Check sheet for the modelled part. Datum: model origin and axes. Units: mm. Face numbers are marked on the shaded views. A direction names the side the tool comes from. Give positions to 0.01 mm unless a question says otherwise; leave off trailing zeros. Order: outer loops, then holes, each group sorted by start corner. A loop starts at its lowest first (then second) coordinate and runs counter-clockwise, first axis right, second up.
Item 1: Sectioned sample at C-C on y = 5. Record the boundary of the cut face in (x, z), and give its area (3 significant figures).
Item 2: Sectioned sample at D-D on x = 7.5. Record the boundary of the cut face in (y, z), and give its area (3 significant figures).
Item 3: Material ranges on line 1 along X through (y, z) = (0, -80); line 2 along X through (y, z) = (0, -74.5); line 3 along Z through (x, y) = (3, 14), recorded low to high.
Item 4: Sectioned sample at A-A on y = 0. Record the boundary of the cut face in (x, z), and give its area (3 significant figures).
Item 5: Release check for a two-part mould opening along Y. For the marked faces 4, 5 and 6 record: released by +Y, released by -Y, zero draft, split by the parting line, or undercut.
Item 6: Gauge pin test, flat ends, axial feed: P1, Ø1, axis at x = 5.5, z = -73.5, coming from the +Y side; P2, Ø3, axis at x = 0.5, z = -78.5, coming from the -Y side; P3, Ø2, axis at x = 12.5, y = 16, coming from the -Z side. Record the tip position at first contact, or that the pin passes through.
Item 7: Access from +Z, -Z, +X, -X, +Y, -Y to the whole of each face (thin tool, end or side, straight path). Record for the marked faces 1, 2 and 3.
Autodesk Inventor part; units mm, degrees
ref_plane "YZ Plane" through (0, 0, 0) normal (1, 0, 0) x (0, 1, 0)
ref_plane "XZ Plane" through (0, 0, 0) normal (0, 1, 0) x (-1, 0, 0)
ref_plane "XY Plane" through (0, 0, 0) normal (0, 0, 1) x (1, 0, 0)
sketch "Sketch1" plane through (0, 0, 0) normal (1, 0, 0) x (0, 1, 0)
  line L0 (0, 0) -> (2.5, 0)
  line L1 (0, 0) -> (4, 0)
  line L2 (2.5, 0) -> (2.5, -7)
  line L3 (2.5, -7) -> (0, -7)
  line L4 (0, -7) -> (20, -7)
  line L5 (4, 0) -> (4, -7)
  line L6 (2.5, -7) -> (2.5, -41)
  line L7 (20, -7) -> (20, -11)
  line L8 (20, -11) -> (2.5, -11)
  line L9 (20, -7) -> (22.5, -7)
  line L10 (22.5, -7) -> (22.5, -11)
  line L11 (22.5, -11) -> (20, -11)
  line L12 (20, -11) -> (20, -7)
  line L13 (20, -7) -> (20, -11)
  line L14 (4, 0) -> (2.5, 0)
  line L15 (2.5, 0) -> (2.5, -11)
  line L16 (2.5, -11) -> (4, -11)
  line L17 (4, -11) -> (4, 0)
  line L18 (2.5, -11) -> (22.5, -11)
  line L19 (22.5, -11) -> (22.5, -7)
  line L20 (22.5, -7) -> (2.5, -7)
  line L21 (2.5, -7) -> (2.5, -11)
  line L22 (2.5, -11) -> (6.5, -11)
  line L23 (0, -7) -> (0, -105.9451)
  line L24 (2.5, -41) -> (25, -41)
  line L25 (0, -82) -> (2.5, -82)
  line L26 (0, -82) -> (4, -82)
  line L27 (2.5, -82) -> (2.5, -75)
  line L28 (2.5, -75) -> (0, -75)
  line L29 (0, -75) -> (20, -75)
  line L30 (4, -82) -> (4, -75)
  line L31 (20, -75) -> (20, -71)
  line L32 (20, -71) -> (2.5, -71)
  line L33 (20, -75) -> (22.5, -75)
  line L34 (22.5, -75) -> (22.5, -71)
  line L35 (22.5, -71) -> (20, -71)
  line L36 (20, -71) -> (20, -75)
  line L37 (20, -75) -> (20, -71)
  line L38 (4, -82) -> (2.5, -82)
  line L39 (2.5, -82) -> (2.5, -71)
  line L40 (2.5, -71) -> (4, -71)
  line L41 (4, -71) -> (4, -82)
  line L42 (2.5, -71) -> (22.5, -71)
  line L43 (22.5, -71) -> (22.5, -75)
  line L44 (22.5, -75) -> (2.5, -75)
  line L45 (2.5, -75) -> (2.5, -71)
  line L46 (2.5, -71) -> (6.5, -71)
  line L47 (2.5, -11) -> (6.5, -11)
  line L48 (6.5, -11) -> (6.5, -71)
  line L49 (6.5, -71) -> (2.5, -71)
  line L50 (2.5, -71) -> (2.5, -11)
  line L51 (6.5, -11) -> (9.5, -11)
  line L52 (9.5, -11) -> (9.5, -14)
  line L53 (9.5, -14) -> (6.5, -14)
  line L54 (6.5, -14) -> (6.5, -11)
  line L55 (6.5, -71) -> (9.5, -71)
  line L56 (9.5, -71) -> (9.5, -68)
  line L57 (9.5, -68) -> (6.5, -68)
  line L58 (6.5, -68) -> (6.5, -71)
  dimension "d1" = 2.5
  dimension "d2" = 4
  dimension "d3" = 7
  dimension "d4" = 20
  dimension "d5" = 34
  dimension "d9" = 4
  dimension "d12" = 2.5
  dimension "d13" = 4
  dimension "d55" = 22.5
  dimension "d56" = 4
  dimension "d80" = 3
  dimension "d81" = 3
  dimension "d82" = 3
  dimension "d83" = 3
revolve "Revolution2" add sketch "Sketch1" angle 360 about axis through (0, 0, -7) along (0, 0, -1) contours L1 L5 L4 L2 | L4 L17 L8 L6 | L4 L7 L8 L17 | L8 L48 L24 L6 | L9 L10 L11 L7 | L24 L48 L32 L50 | L8 L52 L53 L48 | L29 L30 L26 L27 | L39 L32 L41 L29 | L41 L32 L31 L29 | L57 L56 L32 L48 | L31 L35 L34 L33
sketch "Sketch6" plane through (0, 0, 0) normal (0, 1, 0) x (-1, 0, 0)
  line L0 (-2.5, -82) -> (2.5, -82)
  line L1 (0, -82) -> (0, -62)
  line L2 (0, -82) -> (20, -82) construction
  line L3 (0, -65) -> (15, -65) construction
  line L4 (0, -59) -> (15, -59) construction
  line L5 (10.6066, -48.3934) -> (10.6066, -54.3934)
  line L6 (0, -65) -> (0, -59)
  line L7 (0, -62) -> (0, -59.5)
  line L8 (0, -59.5) -> (10.6066, -48.8934)
  line L9 (10.6066, -48.8934) -> (10.6066, -53.8934)
  line L10 (10.6066, -53.8934) -> (0, -64.5)
  line L11 (0, -59.5) -> (0, -64.5)
  point P0 (0, 0)
  dimension "d64" = 20
  dimension "d65" = 90
  dimension "d69" = 15
  dimension "d71" = 15
  dimension "d75" = 2.5
  dimension "d76" = 5
extrude "Extrusion6" cut sketch "Sketch6" along normal mid plane 5
sketch "Sketch7" plane through (0, 0, 0) normal (0, 0, 1) x (1, 0, 0)
  arc A0 (-1.9966, -1.5104) -> (-1.9966, 1.4896) centre (0.0034, -0.0104) ccw
  line L0 (-1.9966, -0.0104) -> (-1.9966, 1.4896)
  line L1 (-1.9966, -0.0104) -> (-1.9966, -1.5104)
  line L2 (-1.9966, 1.4896) -> (-1.9966, -2.007)
  line L3 (-1.9966, -2.007) -> (-3.9862, -2.007)
  line L4 (-3.9862, -2.007) -> (-3.9862, 1.4896)
  line L5 (-3.9862, 1.4896) -> (-1.9966, 1.4896)
  line L6 (-1.9966, -1.5104) -> (-3.2272, -1.5104)
  line L7 (-3.2272, -1.5104) -> (-3.2272, 1.4896)
  line L8 (-3.2272, 1.4896) -> (-1.9966, 1.4896)
  line L9 (-1.9966, 1.4896) -> (-1.9966, -1.5104)
  point P0 (0, 0)
  point P1 (0, 0)
  dimension "d77" = 5
extrude "Extrusion7" add sketch "Sketch7" against normal blind 26 contours L6 L7 L5 L0 L1
sketch "Sketch8" plane through (0, 0, -68) normal (0, 0, 1) x (1, 0, 0)
  arc A0 (0, 2.5) -> (0, -2.5) centre (0, 0) ccw
  circle A1 centre (0, 0) radius 6.5
  point P0 (0, 0)
extrude "Extrusion8" cut sketch "Sketch8" against normal blind 4
sketch "Sketch9" plane through (0, 0, -68) normal (0, 0, 1) x (1, 0, 0)
  circle A0 centre (0, 0) radius 2.5
  circle A1 centre (0, 0) radius 22.5
  point P0 (0, 0)
extrude "Extrusion9" cut sketch "Sketch9" along normal blind 100 contours A0 | A1
sketch "Sketch10" plane through (0, 0, -68) normal (0, 0, 1) x (1, 0, 0)
  circle A0 centre (0, 0) radius 9.5
  circle A1 centre (0, 0) radius 6.5
extrude "Extrusion10" cut sketch "Sketch10" against normal blind 5
properties part number "Spool_revB1"
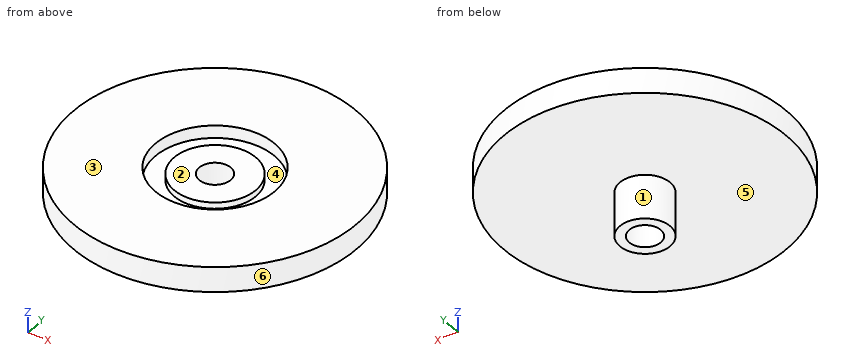
Report:
1. outline: (-21.94, -75) - (21.94, -75) - (21.94, -71) - (8.08, -71) - (8.08, -73) - (4.15, -73) - (4.15, -72) - (-4.15, -72) - (-4.15, -73) - (-8.08, -73) - (-8.08, -71) - (-21.94, -71) - close
1. area: 151 mm2
2. outline: (-21.21, -75) - (21.21, -75) - (21.21, -71) - (5.83, -71) - (5.83, -73) - (-5.83, -73) - (-5.83, -71) - (-21.21, -71) - close
2. area: 146 mm2
3. line 1: x = -4 to -2.5, 2.5 to 4
3. line 2: x = -22.5 to -2.5, 2.5 to 22.5
3. line 3: z = -75 to -71
4. outline: (-22.5, -75) - (-4, -75) - (-4, -82) - (-2.5, -82) - (-2.5, -72) - (-6.5, -72) - (-6.5, -73) - (-9.5, -73) - (-9.5, -71) - (-22.5, -71) - close; (2.5, -82) - (4, -82) - (4, -75) - (22.5, -75) - (22.5, -71) - (9.5, -71) - (9.5, -73) - (6.5, -73) - (6.5, -72) - (2.5, -72) - close
4. area: 161 mm2
5. face 4: undercut
5. face 5: zero draft
5. face 6: split by the parting line
6. P1: stops at y = 21.94
6. P2: stops at y = -4
6. P3: stops at z = -75
7. face 1: -Z
7. face 2: +Z
7. face 3: +Z, +X, -X, +Y, -Y
